```python
from build123d import *

# Parameters (mm, degrees)
ESQUISSE1_R             = 2.5
BOSS_EXTRU_1_DEPTH      = 11
ESQUISSE2_W             = 6.5
ESQUISSE2_H             = 3.5
ENL_V_MAT_EXTRU_1_DEPTH = 7
ESQUISSE3_W             = 6.5
ESQUISSE3_H             = 3.5
ENL_V_MAT_EXTRU_2_DEPTH = 7
ESQUISSE4_R             = 11
ENL_V_MAT_EXTRU_3_DEPTH = 21


with BuildPart() as part:
    # Esquisse1 → Boss.-Extru.1 (new body)
    with BuildSketch(Plane.XY):
        with BuildLine():
            Line((14.875216904, 14.85), (-14.875216904, 14.85))
            ThreePointArc((-14.875216904, 14.85), (-14.933029672, 14.838411285), (-14.981909432, 14.805435784))
            ThreePointArc((-14.981909432, 14.805435784), (-21.063203436, 0), (-14.981909432, -14.805435784))
            ThreePointArc((-14.981909432, -14.805435784), (-14.933029672, -14.838411285), (-14.875216904, -14.85))
            Line((-14.875216904, -14.85), (14.875216904, -14.85))
            ThreePointArc((14.875216904, -14.85), (14.933029672, -14.838411285), (14.981909432, -14.805435784))
            ThreePointArc((14.981909432, -14.805435784), (21.063203436, 0), (14.981909432, 14.805435784))
            ThreePointArc((14.981909432, 14.805435784), (14.933029672, 14.838411285), (14.875216904, 14.85))
        make_face()
        with Locations((-16, 0)):
            Circle(ESQUISSE1_R, mode=Mode.SUBTRACT)
        with Locations((-11.313708499, 11.313708499)):
            Circle(ESQUISSE1_R, mode=Mode.SUBTRACT)
        with Locations((-11.313708499, -11.313708499)):
            Circle(ESQUISSE1_R, mode=Mode.SUBTRACT)
        with Locations((11.313708499, -11.313708499)):
            Circle(ESQUISSE1_R, mode=Mode.SUBTRACT)
        with Locations((16, 0)):
            Circle(ESQUISSE1_R, mode=Mode.SUBTRACT)
        with Locations((11.313708499, 11.313708499)):
            Circle(ESQUISSE1_R, mode=Mode.SUBTRACT)
    extrude(amount=BOSS_EXTRU_1_DEPTH)

    # Esquisse2 → Enlèv. mat.-Extru.1 (cut)
    with BuildSketch(Plane(origin=(0, 14.85, 0), x_dir=(1, 0, 0), z_dir=(0, 1, 0))):
        with Locations((11.313708499, -3.25)):
            Rectangle(ESQUISSE2_W, ESQUISSE2_H)
        with Locations((-11.313708499, -3.25)):
            Rectangle(ESQUISSE2_W, ESQUISSE2_H)
        with Locations((11.313708499, -7.75)):
            Rectangle(ESQUISSE2_W, ESQUISSE2_H)
        with Locations((-11.313708499, -7.75)):
            Rectangle(ESQUISSE2_W, ESQUISSE2_H)
    extrude(amount=-ENL_V_MAT_EXTRU_1_DEPTH, mode=Mode.SUBTRACT)

    # Esquisse3 → Enlèv. mat.-Extru.2 (cut)
    with BuildSketch(Plane.XZ.offset(14.85)):
        with Locations((-11.313708499, 3.25)):
            Rectangle(ESQUISSE3_W, ESQUISSE3_H)
        with Locations((-11.313708499, 7.75)):
            Rectangle(ESQUISSE3_W, ESQUISSE3_H)
        with Locations((11.313708499, 3.25)):
            Rectangle(ESQUISSE3_W, ESQUISSE3_H)
        with Locations((11.313708499, 7.75)):
            Rectangle(ESQUISSE3_W, ESQUISSE3_H)
    extrude(amount=-ENL_V_MAT_EXTRU_2_DEPTH, mode=Mode.SUBTRACT)

    # Esquisse4 → Enlèv. mat.-Extru.3 (cut)
    with BuildSketch(Plane.XY.offset(11)):
        Circle(ESQUISSE4_R)
    extrude(amount=-ENL_V_MAT_EXTRU_3_DEPTH, mode=Mode.SUBTRACT)


solid = part.part
```
Check sheet for the modelled part. Datum: model origin and axes. Units: mm. A direction names the side the tool comes from. Give positions to 0.01 mm unless a question says otherwise; leave off trailing zeros. Order: outer loops, then holes, each group sorted by start corner. A loop starts at its lowest first (then second) coordinate and runs counter-clockwise, first axis right, second up. Notation, with made-up numbers: (15, -29.75) -> (48, -29.75) arc R17 ccw to (48, 0.25) -> close; hole circle Ø9 at (16, -4). An arc over 180 degrees is marked (long way). Use CSV: the item, a comma, the result in double quotes. Start each with the question number.
1) Set-up check for faces 1 (the face through (-12, -14, 1.5)), 2 (the face through (-11.639, 13.792, 10.24)), 3 (the face through (14.564, 11, 3)): record each of +Z, -Z, +X, -X, +Y, -Y from which the full face is reachable in a straight line by a thin tool's end or side.
2) Sectioned sample at B-B, the plane y = 0. Record the boundary of the cut face in (x, z).
3) Go/stop test with flat-tipped pins: P1, Ø1.5, axis at y = 5.5, z = 7, coming from the -X side; P2, Ø4, axis at x = -12, z = 3, coming from the -Y side; P3, Ø1.8, axis at y = 12, z = 7, coming from the -X side; P4, Ø3, axis at y = -9.5, z = 7, coming from the +X side. Record where each tip stops, or that it passes through.
4) Material ranges on line 1 (Z direction, x = -9, y = 12.75); line 2 (X direction, y = -9.5, z = 8.5); line 3 (X direction, y = -13.25, z = 3), recorded low to high. Write a range as from..to.
5) Sectioned sample at D-D, the plane y = -4.75. Record the boundary of the cut face in (x, z), plus the area to 3 significant figures.
6) Sectioned sample at A-A, the plane x = 0. Record the boundary of the cut face in (y, z).
7) Mould release check, pull along Y, two halves, no side actions. Record for faces 4 (the face through (-8.93, -10.56, 5.49)), 5 (the face through (11, 14, 6)), 6 (the face through (-11, -7.85, 8)): released by +Y, released by -Y, zero draft, split by the parting line, or undercut.
8) Sectioned sample at C-C, the plane z = 7.25. Record the boundary of the cut face in (x, y).
Recorded:
1,face 1,"-Y"
1,face 2,"+Z, -Z"
1,face 3,"+Y"
2,outline,"(-21.06, 0) -> (-18.5, 0) -> (-18.5, 11) -> (-21.06, 11) -> close; (-13.5, 0) -> (-11, 0) -> (-11, 11) -> (-13.5, 11) -> close; (11, 0) -> (13.5, 0) -> (13.5, 11) -> (11, 11) -> close; (18.5, 0) -> (21.06, 0) -> (21.06, 11) -> (18.5, 11) -> close"
3,P1,"x = -20.52"
3,P2,"y = -14.85"
3,P3,"x = -17.9"
3,P4,"x = 19.48"
4,line 1,"0..1.5, 5..6, 9.5..11"
4,line 2,"-18.8..-14.56, -8.06..-5.55, 5.55..8.06, 14.56..18.8"
4,line 3,"-16.37..-14.56, -8.06..8.06, 14.56..16.37"
5,outline,"(-20.52, 0) -> (-9.92, 0) -> (-9.92, 11) -> (-20.52, 11) -> close; (9.92, 0) -> (20.52, 0) -> (20.52, 11) -> (9.92, 11) -> close"
5,area,"233 mm2"
6,outline,"(-14.85, 0) -> (-11, 0) -> (-11, 11) -> (-14.85, 11) -> close; (11, 0) -> (14.85, 0) -> (14.85, 11) -> (11, 11) -> close"
7,face 4,"undercut"
7,face 5,"zero draft"
7,face 6,"released by -Y"
8,outline,"(-14.98, -14.81) arc R0.15 ccw to (-14.88, -14.85) -> (-14.56, -14.85) -> (-14.56, -7.85) -> (-8.06, -7.85) -> (-8.06, -14.85) -> (8.06, -14.85) -> (8.06, -7.85) -> (14.56, -7.85) -> (14.56, -14.85) -> (14.88, -14.85) arc R0.15 ccw to (14.98, -14.81) arc R21.06 ccw to (14.98, 14.81) arc R0.15 ccw to (14.88, 14.85) -> (14.56, 14.85) -> (14.56, 7.85) -> (8.06, 7.85) -> (8.06, 14.85) -> (-8.06, 14.85) -> (-8.06, 7.85) -> (-14.56, 7.85) -> (-14.56, 14.85) -> (-14.88, 14.85) arc R0.15 ccw to (-14.98, 14.81) arc R21.06 ccw to start; hole circle Ø5 at (-16, 0); hole circle Ø22 at (0, 0); hole circle Ø5 at (16, 0)"
